For this review, take the finished solid that the model builds, in its own axes (mm). Face numbers are marked on the shaded views. A direction names the side the tool comes from. Give positions to 0.01 mm unless a question says otherwise; leave off trailing zeros. Write each loop counter-clockwise with the first axis right and the second up, starting at its lowest first coordinate (ties: lowest second). Pieces come first, ordered by that corner, then holes. Notation, with made-up numbers: M 38.25,-25 L 77.25,-25 A20 ccw 77.25,-18 Z; hole C 3.5,52 d9. An arc over 180 degrees is marked long. One line per item, written item: value. Start each with the question number.
Item 1: Consider section B-B, the plane z = -6. Write out the cut boundary in (x, y), and give its area (3 significant figures).
Item 2: Tool access review of the marked faces 1, 2, 3 and 4: name each direction out of +Z, -Z, +X, -X, +Y, -Y from which nothing blocks a thin tool from reaching the whole face with its end or side.
Item 3: Consider section C-C, the plane x = -9. Write out the cut boundary in (y, z), and give its area (3 significant figures).
Item 4: Consider section A-A, the plane y = 3.25. Write out the cut boundary in (x, z).
Item 5: Mouldability with a two-part tool opening along Z and no side actions: class the marked faces 5, 6 and 7 as released by +Z, released by -Z, zero draft, split by the parting line, or undercut.
Item 6: Consider section D-D, the plane x = -3.25. Write out the cut boundary in (y, z).
Item 7: Clearance check with flat-ended pins moving along their axes: pin 1 Ø8 at (x, z) = (-15, -13) entering from +Y; pin 2 Ø2 at (y, z) = (6, -12.5) entering from -X; pin 3 Ø1.9 at (y, z) = (2.5, -22) entering from -X; pin 4 Ø1 at (x, y) = (-4, 5) entering from -Z. State where each tip first meets the part, or that it passes through.
Item 8: To check wall thickness, follow probe 1 along Z at (x, y) = (-8.25, 5.25); probe 2 along Z at (x, y) = (-8.2, 0.85); probe 3 along X at (y, z) = (0.7, -15.7). State the ranges of each line that lie inside material, in increasing order.
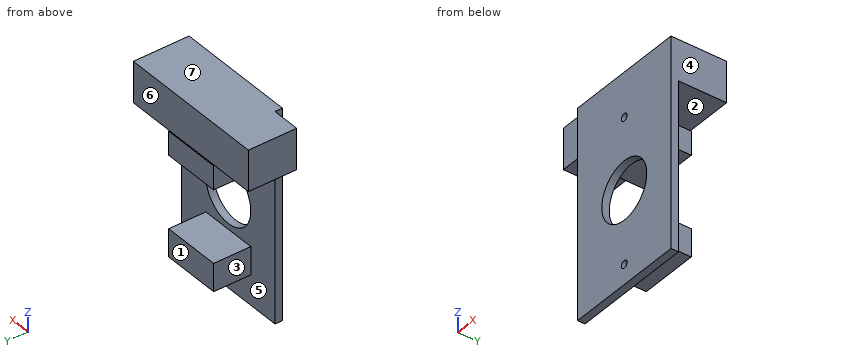
Autodesk Inventor part; units mm, degrees
ref_plane "YZ Plane" through (0, 0, 0) normal (1, 0, 0) x (0, 1, 0)
ref_plane "XZ Plane" through (0, 0, 0) normal (0, 1, 0) x (-1, 0, 0)
ref_plane "XY Plane" through (0, 0, 0) normal (0, 0, 1) x (1, 0, 0)
sketch "Sketch1" plane through (0, 0, 0) normal (0, 1, 0) x (-1, 0, 0)
  line L0 (0, 0) -> (16.4, 0)
  line L1 (16.4, 0) -> (16.4, -28.2)
  line L2 (16.4, -28.2) -> (0, -28.2)
  line L3 (0, -28.2) -> (0, 0)
  dimension "d0" = 16.4
  dimension "d1" = 28.2
extrude "Extrusion1" add sketch "Sketch1" along normal blind 1
sketch "Sketch2" plane through (0, 1, 0) normal (0, 1, 0) x (1, 0, 0)
  circle A0 centre (-8.2, 6) radius 0.5
  circle A1 centre (-8.2, 25.5) radius 0.5
  line L0 (-16.4, 0) -> (0, 0)
  line L1 (-16.4, 28.2) -> (-16.4, 0)
  circle A2 centre (-8.2, 15.7) radius 3.9462
  dimension "d4" = 1
  dimension "d5" = 1
  dimension "d6" = 6
  dimension "d7" = 19.5
  dimension "d8" = 8.2
  dimension "d9" = 8.2
  dimension "d10" = 9.7
  dimension "d11" = 9.8
extrude "Extrusion2" cut sketch "Sketch2" against normal blind 1
sketch "Sketch3" plane through (0, 1, 0) normal (0, 1, 0) x (1, 0, 0)
  line L0 (0, 0) -> (-20.2, 0)
  line L1 (-20.2, 0) -> (-20.2, 5.5)
  line L2 (-20.2, 5.5) -> (0, 5.5)
  line L3 (0, 5.5) -> (0, 0)
  dimension "d14" = 20.2
  dimension "d15" = 5.5
extrude "Extrusion3" add sketch "Sketch3" along normal blind 6.5
sketch "Sketch4" plane through (0, 1, 0) normal (0, 1, 0) x (1, 0, 0)
  line L0 (-8.2, 5.5) -> (0, 5.5)
  line L1 (0, 5.5) -> (0, 28.2)
  line L2 (0, 28.2) -> (-16.4, 28.2)
  line L3 (-16.4, 28.2) -> (-16.4, 5.5)
  line L4 (-16.4, 5.5) -> (-8.2, 5.5)
  circle A0 centre (-8.2, 6) radius 0.5
  circle A1 centre (-8.2, 25.5) radius 0.5
  circle A2 centre (-8.2, 15.7) radius 3.9462
  line L5 (-12.1462, 7.4563) -> (-4.2538, 7.4563)
  line L6 (-4.2538, 7.4563) -> (-4.2538, 10.6519)
  line L7 (-4.2538, 10.6519) -> (-12.1462, 10.6519)
  line L8 (-12.1462, 10.6519) -> (-12.1462, 7.4563)
  line L9 (-12.1462, 24.1585) -> (-4.2538, 24.1585)
  line L10 (-4.2538, 24.1585) -> (-4.2538, 20.409)
  line L11 (-4.2538, 20.409) -> (-12.1462, 20.409)
  line L12 (-12.1462, 20.409) -> (-12.1462, 24.1585)
  point P0 (0, 0)
extrude "Extrusion4" add sketch "Sketch4" along normal blind 5 contours L8 L7 L6 L5 | L9 L10 L11 L12
properties part number "LG_CRD_8521B_Base"
Model answer:
1. outline: M -16.4,0 L -8.7,0 L -8.7,1 L -16.4,1 Z; M -7.7,0 L 0,0 L 0,1 L -7.7,1 Z
1. area: 15.4 mm2
2. face 1: -Z, +X, -X, +Y
2. face 2: +X, -X, +Y
2. face 3: -Z, -X, +Y
2. face 4: +Z, -Z, +X, +Y, -Y
3. outline: M 0,-28.2 L 1,-28.2 L 1,-24.16 L 6,-24.16 L 6,-20.41 L 1,-20.41 L 1,-19.56 L 0,-19.56 Z; M 0,-11.84 L 1,-11.84 L 1,-10.65 L 6,-10.65 L 6,-7.46 L 1,-7.46 L 1,-5.5 L 7.5,-5.5 L 7.5,0 L 0,0 Z
3. area: 90.9 mm2
4. outline: M -20.2,-5.5 L 0,-5.5 L 0,0 L -20.2,0 Z; M -12.15,-24.16 L -4.25,-24.16 L -4.25,-20.41 L -12.15,-20.41 Z; M -12.15,-10.65 L -4.25,-10.65 L -4.25,-7.46 L -12.15,-7.46 Z
5. face 5: undercut
5. face 6: zero draft
5. face 7: released by +Z
6. outline: M 0,-28.2 L 1,-28.2 L 1,-5.5 L 7.5,-5.5 L 7.5,0 L 0,0 Z
7. pin 1: stops at y = 6
7. pin 2: passes through
7. pin 3: stops at x = -12.15
7. pin 4: stops at z = -24.16
8. probe 1: z = -24.16 to -20.41, -10.65 to -7.46, -5.5 to 0
8. probe 2: z = -28.2 to -26, -25 to -19.65, -11.75 to -6.5, -5.5 to 0
8. probe 3: x = -16.4 to -12.15, -4.25 to 0
